```python
from build123d import *

# Parameters (mm, degrees)
SKETCH2_W           = 76.2254
SKETCH2_H           = 58.547
BOSS_EXTRUDE1_DEPTH = 7.62
SKETCH3_W           = 71.1454
SKETCH3_H           = 53.467
CUT_EXTRUDE2_DEPTH  = 3.81
SKETCH4_W           = 5.08
SKETCH4_H           = 5.08
BOSS_EXTRUDE2_DEPTH = 8.7884
CUT_EXTRUDE3_DEPTH  = 5.08


with BuildPart() as part:
    # Sketch2 → Boss-Extrude1 (new body)
    with BuildSketch(Plane(origin=(0, 0, 0), x_dir=(1, 0, 0), z_dir=(0, 1, 0))):
        Rectangle(SKETCH2_W, SKETCH2_H)
    extrude(amount=-BOSS_EXTRUDE1_DEPTH)

    # Sketch3 → Cut-Extrude2 (cut)
    with BuildSketch(Plane(origin=(0, 0, 0), x_dir=(1, 0, 0), z_dir=(0, 1, 0))):
        Rectangle(SKETCH3_W, SKETCH3_H)
    extrude(amount=-CUT_EXTRUDE2_DEPTH, mode=Mode.SUBTRACT)

    # Sketch4 → Boss-Extrude2 (add)
    with BuildSketch(Plane.XZ.offset(7.62)):
        with Locations((-29.8577, 21.0185)):
            Rectangle(SKETCH4_W, SKETCH4_H)
        with Locations((29.8577, 21.0185)):
            Rectangle(SKETCH4_W, SKETCH4_H)
    boss_extrude2 = extrude(amount=BOSS_EXTRUDE2_DEPTH)

    # Sketch5 → Cut-Extrude3 (cut)
    with BuildSketch(Plane.XY.offset(23.5585)):
        Polygon((29.8577, -16.4084), (27.3177, -16.4084), (27.3177, -12.606876095), align=None)
        Polygon((-29.8577, -16.4084), (-32.3977, -12.606876095), (-32.3977, -16.4084), align=None)
        Polygon((27.3177, -7.62), (27.3177, -11.336876095), (29.038774553, -10.798216701), (29.038774553, -7.62), align=None)
        Polygon((-32.3977, -11.336876095), (-30.676625447, -10.798216701), (-30.676625447, -7.62), (-32.3977, -7.62), align=None)
    cut_extrude3 = extrude(amount=-CUT_EXTRUDE3_DEPTH, mode=Mode.SUBTRACT)

    # Mirror1: Boss-Extrude2, Cut-Extrude3 across plane
    add(boss_extrude2.mirror(Plane.XY))
    add(cut_extrude3.mirror(Plane.XY), mode=Mode.SUBTRACT)


solid = part.part
```
Design review of the part built by this model. Coordinates are the model's own, in mm. A direction names the side the tool comes from. Round coordinates to 2 decimals unless told otherwise and drop trailing zeros. Write each loop counter-clockwise with the first axis right and the second up, starting at its lowest first coordinate (ties: lowest second). Pieces come first, ordered by that corner, then holes.
Item 1: We need section D-D on z = -11.5. Write out the cut boundary in (x, y), and give its area (3 significant figures).
Item 2: We need section A-A on y = -8.5. Write out the cut boundary in (x, z), and give its area (3 significant figures).
Item 3: We need section C-C on z = -21.5. Write out the cut boundary in (x, y), and give its area (3 significant figures).
Item 4: Clearance check with flat-ended pins moving along their axes: pin 1 Ø2.5 at (y, z) = (-13, 20.5) entering from +X; pin 2 Ø1.5 at (x, y) = (30.5, -11.5) entering from +Z; pin 3 Ø1.5 at (x, y) = (-28.5, -10) entering from -Z. State where each tip first meets the part, or that it passes through.
Item 5: For probe 1 along Z at (x, y) = (15, -3.5); probe 2 along X at (y, z) = (-0.75, -20); probe 3 along Z at (x, y) = (-28, -10.5), list the stretches that pass through material, from the lowest coordinate up.
Item 6: The part is to be moulded in two halves that separate along Z. For faces 4 (the flat face through (-29, -12, -23.558)), 5 (the flat face through (-31.11, -14.534, 21.054)), 6 (the flat face through (30, -12, 23.558)), 7 (the flat face through (30, -12, 18.478)), say which applies: +Z half, -Z half, draft (parallel to the pull), parting line (faces both ways), or undercut.
Item 7: For faces 1 (the flat face through (-30.677, -9, 21)), 2 (the flat face through (-29, -12, -18.478)), 3 (the flat face through (0, -2, -26.734)), list the 3-axis set-ups (+Z, -Z, +X, -X, +Y, -Y) from which the entire face can be reached by the end or side of a thin tool; tool diameter is ignored.
Item 8: We need section B-B on x = -26.5. Write out the cut boundary in (y, z), and give its area (3 significant figures).
Returned:
1. outline: (-38.11, -7.62) - (38.11, -7.62) - (38.11, 0) - (35.57, 0) - (35.57, -3.81) - (-35.57, -3.81) - (-35.57, 0) - (-38.11, 0) - close
1. area: 310 mm2
2. outline: (-30.68, -23.56) - (-27.32, -23.56) - (-27.32, -18.48) - (-30.68, -18.48) - close; (-30.68, 18.48) - (-27.32, 18.48) - (-27.32, 23.56) - (-30.68, 23.56) - close; (29.04, -23.56) - (32.4, -23.56) - (32.4, -18.48) - (29.04, -18.48) - close; (29.04, 18.48) - (32.4, 18.48) - (32.4, 23.56) - (29.04, 23.56) - close
2. area: 68.3 mm2
3. outline: (-38.11, -7.62) - (-30.68, -7.62) - (-30.68, -10.8) - (-32.4, -11.34) - (-32.4, -12.61) - (-29.86, -16.41) - (-27.32, -16.41) - (-27.32, -7.62) - (29.04, -7.62) - (29.04, -10.8) - (27.32, -11.34) - (27.32, -12.61) - (29.86, -16.41) - (32.4, -16.41) - (32.4, -7.62) - (38.11, -7.62) - (38.11, 0) - (35.57, 0) - (35.57, -3.81) - (-35.57, -3.81) - (-35.57, 0) - (-38.11, 0) - close
3. area: 378 mm2
4. pin 1: stops at x = 32.4
4. pin 2: stops at z = 23.56
4. pin 3: stops at z = -23.56
5. probe 1: z = -29.27 to -26.73, 26.73 to 29.27
5. probe 2: x = -38.11 to -35.57, 35.57 to 38.11
5. probe 3: z = -23.56 to -18.48, 18.48 to 23.56
6. face 4: -Z half
6. face 5: draft
6. face 6: +Z half
6. face 7: undercut
7. face 1: +Z, -Z, -X
7. face 2: +X, -X, -Y
7. face 3: +Y
8. outline: (-7.62, -29.27) - (0, -29.27) - (0, -26.73) - (-3.81, -26.73) - (-3.81, 26.73) - (0, 26.73) - (0, 29.27) - (-7.62, 29.27) - close
8. area: 242 mm2
